For this review, take the finished solid that the model builds, in its own axes (mm). Face numbers are marked on the shaded views. A direction names the side the tool comes from. Round coordinates to 2 decimals unless told otherwise and drop trailing zeros. Order: outer loops, then holes, each group sorted by start corner. A loop starts at its lowest first (then second) coordinate and runs counter-clockwise, first axis right, second up. Notation, with made-up numbers: M 38.25,-40 L 93.25,-40 A7 cw 93.25,-30 Z; hole C 67,83.25 d7. An arc over 180 degrees is marked long. Write item = value, one per line. Start each with the question number.
from build123d import *

# Parameters (mm, degrees)
PAD099_DEPTH    = 1
SKETCH286_R     = 0.95
PAD100_DEPTH    = 2.5
PAD101_DEPTH    = 1.5
SKETCH288_W     = 8.5
SKETCH288_H     = 5.6
PAD102_DEPTH    = 5.2
SKETCH289_R     = 1.5
POCKET169_DEPTH = 15
FILLET002_R     = 6
FILLET004_R     = 2


with BuildPart() as part:
    # Sketch277 → Pad099 (new body)
    with BuildSketch(Plane.YZ.offset(57.2)):
        Polygon((-20, 2.8), (-20, -2.8), (-6, -10.3), (0, -10.3), (0, 10.3), (-6, 10.3), align=None)
    pad099 = extrude(amount=PAD099_DEPTH)

    # Sketch286 (on Face7 of Pad099) → Pad100 (join)
    with BuildSketch(Plane(origin=(57.2, 0, 0), x_dir=(0, 1, 0), z_dir=(-1, 0, 0))):
        with Locations((-6, 0)):
            Circle(SKETCH286_R)
    pad100 = extrude(amount=PAD100_DEPTH)

    # Sketch287 (on Face4 of Pad100) → Pad101 (join)
    with BuildSketch(Plane(origin=(57.2, 0, 0), x_dir=(0, 1, 0), z_dir=(-1, 0, 0))):
        with BuildLine():
            Line((-20, -2.8), (-20, 2.8))
            Line((-20, 2.8), (-6, 10.3))
            Line((-6, 10.3), (0, 10.3))
            Line((0, 9.1), (0, 10.3))
            ThreePointArc((0, 9.1), (-9.1, 0), (0, -9.1))
            Line((0, -9.1), (0, -10.3))
            ThreePointArc((-9.9121138008, -2.8), (-6.2149014473, -8.2137080542), (0, -10.3))
            Line((-20, -2.8), (-9.9121138008, -2.8))
        make_face()
    pad101 = extrude(amount=PAD101_DEPTH)

    # Sketch288 (on Face18 of Pad101) → Pad102 (join)
    with BuildSketch(Plane(origin=(57.2, 0, 0), x_dir=(0, 1, 0), z_dir=(-1, 0, 0))):
        with Locations((-15.65, 0)):
            Rectangle(SKETCH288_W, SKETCH288_H)
    pad102 = extrude(amount=PAD102_DEPTH)

    # Sketch289 (on Face5 of Pad102) → Pocket169 (cut, symmetric)
    with BuildSketch(Plane.YZ.offset(58.2)):
        with Locations((-15, 0)):
            Circle(SKETCH289_R)
    pocket169 = extrude(amount=POCKET169_DEPTH, both=True, mode=Mode.SUBTRACT)

    # Mirrored011: Pad099, Pad100, Pad101, Pad102, Pocket169 across Sketch277 V_Axis
    add(pad099.mirror(Plane(origin=(57.2, 0, 0), x_dir=(1, 0, 0), z_dir=(0, 1, 0))))
    add(pad100.mirror(Plane(origin=(57.2, 0, 0), x_dir=(1, 0, 0), z_dir=(0, 1, 0))))
    add(pad101.mirror(Plane(origin=(57.2, 0, 0), x_dir=(1, 0, 0), z_dir=(0, 1, 0))))
    add(pad102.mirror(Plane(origin=(57.2, 0, 0), x_dir=(1, 0, 0), z_dir=(0, 1, 0))))
    add(pocket169.mirror(Plane(origin=(57.2, 0, 0), x_dir=(1, 0, 0), z_dir=(0, 1, 0))), mode=Mode.SUBTRACT)

    # Fillet002
    fillet002_edges = [part.edges().sort_by_distance(p)[0] for p in [
        (57.7, -6, -10.3),
        (56.45, -6, -10.3),
        (57.7, 6, -10.3),
        (56.45, 6, -10.3),
        (57.7, -6, 10.3),
        (57.7, 6, 10.3),
    ]]
    fillet(fillet002_edges, radius=FILLET002_R)

    # Fillet004
    fillet004_edges = [part.edges().sort_by_distance(p)[0] for p in [
        (53.85, 11.4, -2.8),
        (53.85, -11.4, -2.8),
    ]]
    fillet(fillet004_edges, radius=FILLET004_R)


solid = part.part
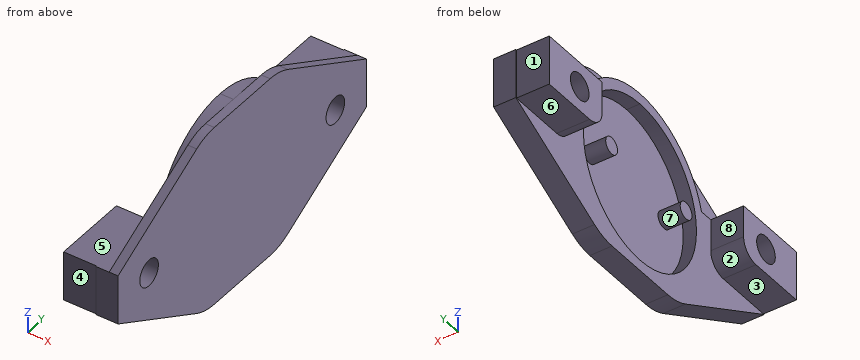
(1) For the marked faces 4, 5, 6, 7 and 8, list the 3-axis set-ups (+Z, -Z, +X, -X, +Y, -Y) from which the entire face can be reached by the end or side of a thin tool; tool diameter is ignored.
(2) Draft analysis for pull direction Y (two halves, no side actions). For the marked faces 1, 2 and 3, state which applies: released by +Y, released by -Y, zero draft, split by the parting line, or undercut.
(3) We need section D-D, the plane y = 15. Write out the cut boundary in (x, z), then the cut area to 3 significant figures.
(4) For line 1 along Y through (x, z) = (55.5, 2); line 2 along Z through (x, y) = (54.25, 15); line 3 along X through (y, z) = (-4.5, 1.75), list the stretches that pass through material, from the lowest coordinate up.
(5) We need section B-B, the plane z = 0. State how many separate pieces and enclosed holes the cut face has, then the cut area to 3 significant figures.
(6) We need section A-A, the plane x = 54. Write out the cut boundary in (y, z).
(7) We need section C-C, the plane x = 56.25. Write out the cut boundary in (y, z), then the cut area to 3 significant figures.
(8) Insertion check: pin 1 (1.1 mm diameter, centred on x = 53, y = -17, fed in from -Z); pin 2 (1.1 mm diameter, centred on x = 54.5, z = 1, fed in from -Y); pin 3 (3 mm diameter, centred on x = 53.5, z = 0.5, fed in from +Y); pin 4 (5 mm diameter, centred on y = 15, z = 0, fed in from +X). Each pin has a flat end and moves straight along its axis. Give the tip position at first contact, or say it passes through.
Values:
q1.face_4 = +Z, -Z, -X, -Y
q1.face_5 = +Z, -X, -Y
q1.face_6 = -Z, -X, +Y, -Y
q1.face_7 = -X
q1.face_8 = +Z, -Z, -X
q2.face_1 = released by +Y
q2.face_2 = undercut
q2.face_3 = zero draft
q3.outline = M 52,-2.8 L 55.7,-2.8 L 55.7,-5.48 L 58.2,-5.48 L 58.2,-1.5 L 52,-1.5 Z; M 52,1.5 L 58.2,1.5 L 58.2,5.48 L 57.2,5.48 L 57.2,2.8 L 52,2.8 Z
q3.area = 25.5 mm²
q4.line_1 = -19.9 to -11.4, 11.4 to 19.9
q4.line_2 = -2.8 to -1.5, 1.5 to 2.8
q4.line_3 = 57.2 to 58.2
q5.separate_pieces = 3
q5.enclosed_holes = 0
q5.area = 108 mm²
q6.outline = M -19.9,-2.8 L -13.4,-2.8 A2 ccw -11.4,-0.8 L -11.4,2.8 L -19.9,2.8 Z; M 11.4,-0.8 A2 ccw 13.4,-2.8 L 19.9,-2.8 L 19.9,2.8 L 11.4,2.8 Z; hole C -15,0 d3; hole C 15,0 d3
q7.outline = M -20,-2.8 L -7.33,-9.59 A6 ccw -4.49,-10.3 L 4.49,-10.3 A6 ccw 7.33,-9.59 L 20,-2.8 L 20,2.8 L 9.91,2.8 A10.3 ccw -9.91,2.8 L -20,2.8 Z; C -6,0 d1.9; C 6,0 d1.9; hole C -15,0 d3; hole C 0,0 d18.2; hole C 15,0 d3
q7.area = 260 mm²
q8.pin_1 = -2.8
q8.pin_2 = -19.9
q8.pin_3 = 19.9
q8.pin_4 = 58.2
